Geometry: final body of the model. Coordinates: model frame, mm. A direction names the side the tool comes from. Coordinates: 2 decimals unless noted, no trailing zeros. Write each loop counter-clockwise with the first axis right and the second up, starting at its lowest first coordinate (ties: lowest second). Pieces come first, ordered by that corner, then holes. Notation, with made-up numbers: (66.5, -25) - (102.5, -25) arc R15 ccw to (102.5, 3) - close; hole circle Ø9 at (33.25, -22.5). An arc over 180 degrees is marked (long way). Answer as a JSON object with one key per item and string values. Group by question number.
Item 1: Section C-C on x = 0. Return loops of the section in (y, z), and give its area (3 significant figures).
Item 2: Section D-D on x = 31. Return loops of the section in (y, z).
Item 3: Set-up query: faces 4 (the flat face through (-8, 0, -1)), 5 (the cylindrical face through (7.84, 1.521, 7.716)). Return all of +Z, -Z, +X, -X, +Y, -Y with unobstructed straight access to the full face (end or side cutting, diameter ignored); none if empty.
Item 4: First-contact query: pin 1 Ø1 at (y, z) = (1, 25) entering from +X; pin 2 Ø2.5 at (x, z) = (0, -8) entering from -Y; pin 3 Ø1.5 at (x, y) = (-9.5, 2) entering from -Z. Flat tips, straight axial feed; report the tip coordinate or a pass-through.
Item 5: Section B-B on y = 1.2. Return loops of the section in (x, z).
Item 6: Mould query, pull axis X, two halves, no side actions, for faces 1 (the cylindrical face through (-7.716, 1.521, 7.84)), 2 (the flat face through (-8, 3, -1)), 3 (the cylindrical face through (-39.05, 1.48, -8.67)). Classes: pulls with the +X half, pulls with the -X half, needs draft (parallel to the pull), parting line crosses it, or undercut.
Item 7: Line query: line 1 along X through (y, z) = (1.15, 0); line 2 along Z through (x, y) = (-28.5, 1); line 3 along X through (y, z) = (1.65, -8). Output: solid intervals per line, ascending. Write a range as from..to.
Item 8: Section A-A on z = 0. Return loops of the section in (x, y), and give its area (3 significant figures).
```python
from build123d import *

# Parameters (mm, degrees)
SKETCH_1_R          = 40
SKETCH_1_R_2        = 1.55
EXTRUDE_1_DEPTH     = 3
SKETCH_5_R          = 2.1
CUT_EXTRUDE_4_DEPTH = 10
CUT_EXTRUDE_5_DEPTH = 10


with BuildPart() as part:
    # 草图1 → 凸台-拉伸1 (new body)
    with BuildSketch(Plane(origin=(0, 0, 0), x_dir=(1, 0, 0), z_dir=(0, 1, 0))):
        with Locations(Location((0, 0, 0), (0, 0, 270))):
            Circle(SKETCH_1_R)
        with Locations(Location((0, 8, 0), (0, 0, 270))):
            Circle(SKETCH_1_R_2, mode=Mode.SUBTRACT)
        with Locations(Location((0, -8, 0), (0, 0, 270))):
            Circle(SKETCH_1_R_2, mode=Mode.SUBTRACT)
    extrude(amount=EXTRUDE_1_DEPTH)

    # 草图5 → 切除-拉伸4 (cut)
    with BuildSketch(Plane(origin=(0, 3, 0), x_dir=(1, 0, 0), z_dir=(0, 1, 0))):
        with Locations(Location((0, 0, 0), (0, 0, 270))):
            Circle(SKETCH_5_R)
    extrude(amount=-CUT_EXTRUDE_4_DEPTH, mode=Mode.SUBTRACT)

    # 草图4 → 切除-拉伸5 (cut)
    with BuildSketch(Plane(origin=(0, 3, 0), x_dir=(1, 0, 0), z_dir=(0, 1, 0))):
        with BuildLine():
            Line((-5.199210429, 9.693720179), (-5.286154205, 32.573863353))
            ThreePointArc((-5.286154205, 32.573863353), (-23.423025076, 23.245685542), (-32.613096487, 5.038445946))
            Line((-32.613096487, 5.038445946), (-9.732953313, 5.125389722))
            ThreePointArc((-9.732953313, 5.125389722), (-7.807675025, 7.748561847), (-5.199210429, 9.693720179))
        make_face()
        with BuildLine():
            ThreePointArc((32.573863353, 5.286154205), (23.245685542, 23.423025076), (5.038445946, 32.613096487))
            Line((5.038445946, 32.613096487), (5.125389722, 9.732953313))
            ThreePointArc((5.125389722, 9.732953313), (7.748561847, 7.807675025), (9.693720179, 5.199210429))
            Line((9.693720179, 5.199210429), (32.573863353, 5.286154205))
        make_face()
        with BuildLine():
            ThreePointArc((5.286154205, -32.573863353), (23.423025076, -23.245685542), (32.613096487, -5.038445946))
            Line((32.613096487, -5.038445946), (9.732953313, -5.125389722))
            ThreePointArc((9.732953313, -5.125389722), (7.807675025, -7.748561847), (5.199210429, -9.693720179))
            Line((5.199210429, -9.693720179), (5.286154205, -32.573863353))
        make_face()
        with BuildLine():
            Line((-9.693720179, -5.199210429), (-32.573863353, -5.286154205))
            ThreePointArc((-32.573863353, -5.286154205), (-23.245685542, -23.423025076), (-5.038445946, -32.613096487))
            Line((-5.038445946, -32.613096487), (-5.125389722, -9.732953313))
            ThreePointArc((-5.125389722, -9.732953313), (-7.748561847, -7.807675025), (-9.693720179, -5.199210429))
        make_face()
    extrude(amount=-CUT_EXTRUDE_5_DEPTH, mode=Mode.SUBTRACT)


solid = part.part
```
Checks:
{
 "1": {"outline": "(0, -40) - (3, -40) - (3, -9.55) - (0, -9.55) - close; (0, -6.45) - (3, -6.45) - (3, -2.1) - (0, -2.1) - close; (0, 2.1) - (3, 2.1) - (3, 6.45) - (0, 6.45) - close; (0, 9.55) - (3, 9.55) - (3, 40) - (0, 40) - close", "area": "209 mm^2"},
 "2": {"outline": "(0, -25.28) - (3, -25.28) - (3, -11.31) - (0, -11.31) - close; (0, -5.28) - (3, -5.28) - (3, 5.04) - (0, 5.04) - close; (0, 11.31) - (3, 11.31) - (3, 25.28) - (0, 25.28) - close"},
 "3": {"face 4": "+Z, -Z, +X, -X, -Y", "face 5": "+Y, -Y"},
 "4": {"pin 1": "x = 31.62", "pin 2": "through", "pin 3": "z = -39.03"},
 "5": {"outline": "circle Ø80 at (0, 0); hole (-32.61, -5.04) arc R33 ccw to (-5.29, -32.57) - (-5.2, -9.69) arc R11 cw to (-9.73, -5.13) - close; hole (-32.57, 5.29) - (-9.69, 5.2) arc R11 cw to (-5.13, 9.73) - (-5.04, 32.61) arc R33 ccw to start; hole circle Ø4.2 at (0, 0); hole circle Ø3.1 at (0, -8); hole circle Ø3.1 at (0, 8); hole (5.04, -32.61) arc R33 ccw to (32.57, -5.29) - (9.69, -5.2) arc R11 cw to (5.13, -9.73) - close; hole (5.2, 9.69) arc R11 cw to (9.73, 5.13) - (32.61, 5.04) arc R33 ccw to (5.29, 32.57) - close"},
 "6": {"face 1": "undercut", "face 2": "needs draft", "face 3": "parting line crosses it"},
 "7": {"line 1": "-40..-2.1, 2.1..40", "line 2": "-28.07..-16.64, -5.05..5.27, 16.64..28.07", "line 3": "-39.19..-32.02, -7.55..-1.55, 1.55..7.55, 32.02..39.19"},
 "8": {"outline": "(-40, 0) - (-2.1, 0) - (-2.1, 3) - (-40, 3) - close; (2.1, 0) - (40, 0) - (40, 3) - (2.1, 3) - close", "area": "227 mm^2"}
}
